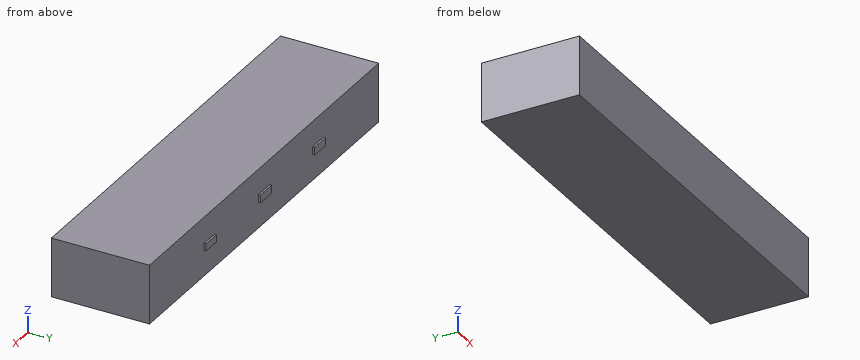
```python
from build123d import *

# Parameters (mm, degrees)
F0_W     = 63.5
F0_H     = 38.1
F1_DEPTH = 132.08
F2_W     = 12.192
F2_H     = 4.572
F3_DEPTH = 1.27


with BuildPart() as f1:
    # F0 (on Right) → F1 (new body, symmetric)
    with BuildSketch(Plane.YZ):
        Rectangle(F0_W, F0_H)
    extrude(amount=F1_DEPTH, both=True)

    # F2 (on face) → F3 (join)
    with BuildSketch(Plane(origin=(0, 31.75, 0), x_dir=(-1, 0, 0), z_dir=(0, 1, 0))):
        with Locations((-63.034566, -0.225544)):
            Rectangle(F2_W, F2_H)
        Polygon((-6.334301, 2.060456), (-6.334301, -2.511544), (6.365699, -2.511544), (6.365699, 2.568456), (5.857699, 2.568456), (-6.334301, 2.568456), align=None)
        Polygon((68.733813, -2.511544), (68.733813, 2.568456), (68.225813, 2.568456), (56.033813, 2.568456), (56.033813, 2.060456), (56.033813, -2.511544), align=None)
    extrude(amount=F3_DEPTH)


solid = f1.part
```
Input: part model. Units: mm. Frame: model coordinates. Give positions to 0.01 mm unless a question says otherwise; leave off trailing zeros. Order: outer loops, then holes, each group sorted by start corner. A loop starts at its lowest first (then second) coordinate and runs counter-clockwise, first axis right, second up.
1. Material intervals for L1, parallel to Y at x = -18, z = -15, sorted ascending.
Derived:
L1: y = -31.75 to 31.75
2. Pin query (flat end, axial travel): pin 1 (0.6 mm diameter, centred on y = 32.5, z = 1, fed in from -X); pin 2 (0.6 mm diameter, centred on x = -65, y = 32.5, fed in from +Z); pin 3 (1 mm diameter, centred on y = 32.5, z = 0, fed in from +X); pin 4 (1.4 mm diameter, centred on y = 32, z = 1, fed in from -X). Return the tip coordinate at first contact, or that it passes through.
Derived:
pin 1: stops at x = -68.73
pin 2: stops at z = 2.57
pin 3: stops at x = 69.13
pin 4: stops at x = -132.08
3. Section A-A on x = -44. Return the cut outline in (y, z).
Derived:
outline: (-31.75, -19.05) - (31.75, -19.05) - (31.75, 19.05) - (-31.75, 19.05) - close
4. Section B-B on z = -9.5. Return the cut outline in (x, y).
Derived:
outline: (-132.08, -31.75) - (132.08, -31.75) - (132.08, 31.75) - (-132.08, 31.75) - close
